The drawing under review shows one solid part. Ordinate dimensions are in mm from its lowest x, y, z. A direction names the side the tool comes from. Round coordinates to 2 decimals unless told otherwise and drop trailing zeros. Order: outer loops, then holes, each group sorted by start corner. A loop starts at its lowest first (then second) coordinate and runs counter-clockwise, first axis right, second up. Notation, with made-up numbers: M 63.25,-12 L 95.25,-12 A18 cw 95.25,12 Z; hole C 29.5,51 d5. An arc over 180 degrees is marked long. Answer as a JSON object with one key per item and string values. Group by question number.
1. Add section D-D on z = 55. State the section outline as (x, y) points.
2. Mouldability with a two-part tool opening along X and no side actions: class the marked faces 3, 4 and 5 as released by +X, released by -X, zero draft, split by the parting line, or undercut.
3. Add section A-A on z = 77.5. State the section outline as (x, y) points, and give its area (3 significant figures).
4. Add section C-C on y = 20. State the section outline as (x, z) points.
5. To check wall thickness, follow probe 1 along Z at (x, y) = (182, 45); probe 2 along X at (y, z) = (39, 60); probe 3 along X at (y, z) = (5, 57.5). State the ranges of each line that lie inside material, in increasing order. Write a range as [from, to].
6. Machinability: for the marked faces 1 and 2, which of the approach directions +Z, -Z, +X, -X, +Y, -Y give a long, thin tool a straight path to every point of the face, cutting with its end or side? Answer none if there is none.
7. Add section B-B on x = 168. State the section outline as (y, z) points.
8. Clearance check with a flat-ended pin moving along its axis: P1, Ø3, axis at x = 32.5, y = 38, coming from the +Z side. State where the tip first meets the part, or that it passes through.
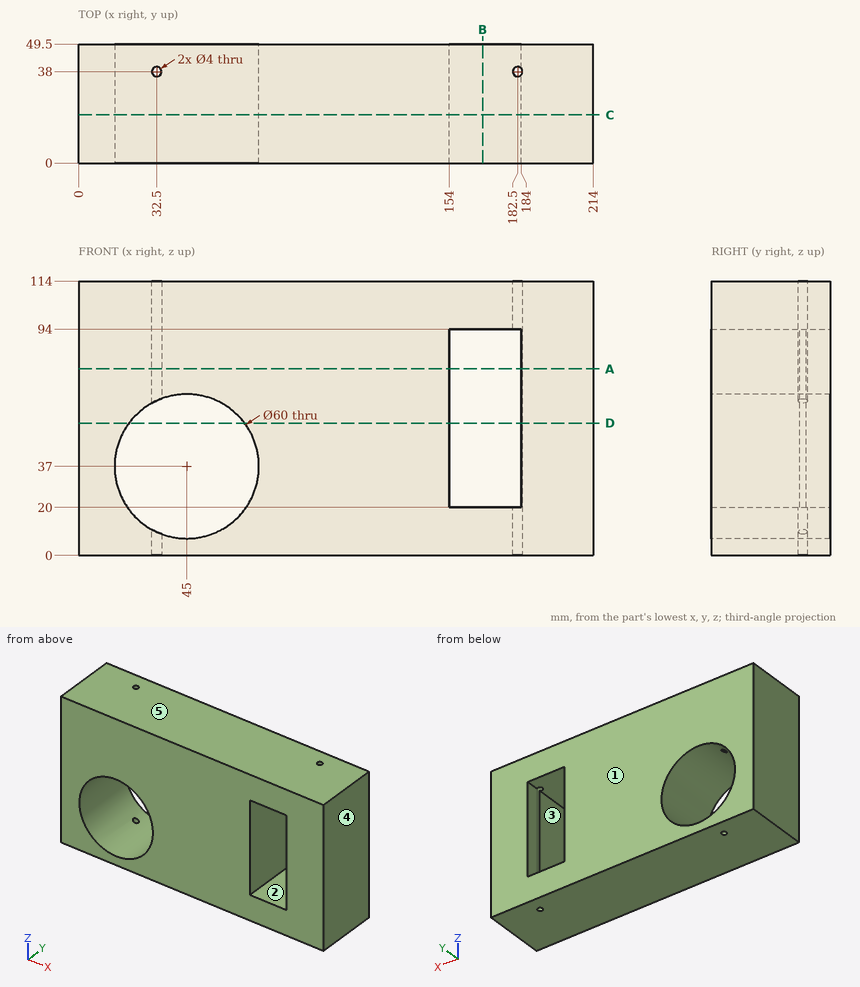
Recorded:
{
 "1": {"outline": "M 0,0 L 21,0 L 21,49.5 L 0,49.5 Z; M 69,0 L 154,0 L 154,49.5 L 69,49.5 Z; M 184,0 L 214,0 L 214,49.5 L 184,49.5 L 184,39.32 A2 cw 184,36.68 Z"},
 "2": {"face 3": "undercut", "face 4": "released by +X", "face 5": "zero draft"},
 "3": {"outline": "M 0,0 L 154,0 L 154,49.5 L 0,49.5 Z; M 184,0 L 214,0 L 214,49.5 L 184,49.5 L 184,39.32 A2 cw 184,36.68 Z; hole C 32.5,38 d4", "area": "9,090 mm²"},
 "4": {"outline": "M 0,0 L 214,0 L 214,114 L 0,114 Z; hole C 45,37 d60; hole M 154,20 L 184,20 L 184,94 L 154,94 Z"},
 "5": {"probe 1": "z = [0, 20], [94, 114]", "probe 2": "x = [0, 25.74], [64.26, 154], [184.23, 214]", "probe 3": "x = [0, 23.1], [66.9, 154], [184, 214]"},
 "6": {"face 1": "+Z, -Z, +X, -X, +Y", "face 2": "+Y, -Y"},
 "7": {"outline": "M 0,0 L 49.5,0 L 49.5,20 L 0,20 Z; M 0,94 L 49.5,94 L 49.5,114 L 0,114 Z"},
 "8": {"P1": "passes through"}
}
